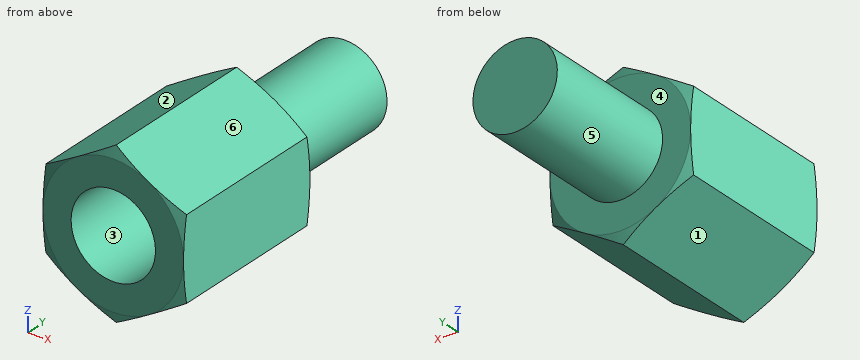
```python
from build123d import *

# Parameters (mm, degrees)
SKETCH1_R                = 1.5
BOSS_EXTRUDE1_DEPTH      = 6
BOSS_EXTRUDE2_DEPTH      = 5
BOSS_EXTRUDE2_DEPTH_BACK = 1.5
SKETCH7_R                = 1.5


with BuildPart() as part:
    # Sketch1 → Boss-Extrude1 (new body)
    with BuildSketch(Plane(origin=(0, 0, 0), x_dir=(1, 0, 0), z_dir=(0, 1, 0))):
        Polygon((0, 2.886751346), (-2.5, 1.443375673), (-2.5, -1.443375673), (0, -2.886751346), (2.5, -1.443375673), (2.5, 1.443375673), align=None)
        with Locations(Location((0, 0, 0), (0, 0, 270))):
            Circle(SKETCH1_R, mode=Mode.SUBTRACT)
    extrude(amount=BOSS_EXTRUDE1_DEPTH)

    # Sketch6 → Cut-Revolve1 (revolve, cut)
    with BuildSketch(Plane.ZY):
        Polygon((2.5, 6), (2.886751346, 6), (2.886751346, 5.859234022), align=None)
    cut_revolve1 = revolve(axis=Axis((0, 6, 0), (0, 1, 0)), mode=Mode.SUBTRACT)

    # Mirror1: Cut-Revolve1 across plane
    add(cut_revolve1.mirror(Plane.ZX.offset(3)), mode=Mode.SUBTRACT)

    # Sketch7 → Boss-Extrude2 (add, two sides: drawn at the far end of the back side and taken through both)
    with BuildSketch(Plane(origin=(0, 6, 0), x_dir=(1, 0, 0), z_dir=(0, 1, 0)).offset(-BOSS_EXTRUDE2_DEPTH_BACK)):
        with Locations(Location((0, 0, 0), (0, 0, 270))):
            Circle(SKETCH7_R)
    extrude(amount=BOSS_EXTRUDE2_DEPTH + BOSS_EXTRUDE2_DEPTH_BACK)


solid = part.part
```
Check sheet for the modelled part. Datum: model origin and axes. Units: mm. Face numbers are marked on the shaded views. A direction names the side the tool comes from. Round coordinates to 2 decimals unless told otherwise and drop trailing zeros. Order: outer loops, then holes, each group sorted by start corner. A loop starts at its lowest first (then second) coordinate and runs counter-clockwise, first axis right, second up.
1) Section check B-B (y = 8). Record the boundary of the cut face in (x, z).
2) Go/stop test with flat-tipped pins: pin 1 Ø1.5 at (x, z) = (0.5, -0.5) entering from -Y; pin 2 Ø1 at (x, z) = (-1.5, -1.5) entering from +Y; pin 3 Ø3 at (y, z) = (9.5, 0) entering from +X. Record where each tip stops, or that it passes through.
3) Tool access check on the marked faces 5 and 6. Record the directions out of +Z, -Z, +X, -X, +Y, -Y that give a thin tool (end or side, any length) a straight path to the whole face; none if there is none.
4) Mould release check, pull along Z, two halves, no side actions. Record for the marked faces 1, 2, 3 and 4: +Z half, -Z half, draft (parallel to the pull), parting line (faces both ways), or undercut.
5) Section check A-A (y = 2.5). Record the boundary of the cut face in (x, z), and give its area (3 significant figures).
6) Scan lines: line 1 (Y direction, x = -2, z = 1.2); line 2 (Y direction, x = 0.9, z = 0.95); line 3 (Z direction, x = 0.05, y = 10). Record each from-to range of solid material in increasing order.
Result:
1. outline: circle Ø3 at (0, 0)
2. pin 1: stops at y = 4.5
2. pin 2: stops at y = 6
2. pin 3: stops at x = 1.5
3. face 5: +Y
3. face 6: +Z, +X, +Y, -Y
4. face 1: -Z half
4. face 2: +Z half
4. face 3: undercut
4. face 4: draft
5. outline: (-2.5, -1.44) - (0, -2.89) - (2.5, -1.44) - (2.5, 1.44) - (0, 2.89) - (-2.5, 1.44) - close; hole circle Ø3 at (0, 0)
5. area: 14.6 mm2
6. line 1: y = 0 to 6
6. line 2: y = 4.5 to 11
6. line 3: z = -1.5 to 1.5
